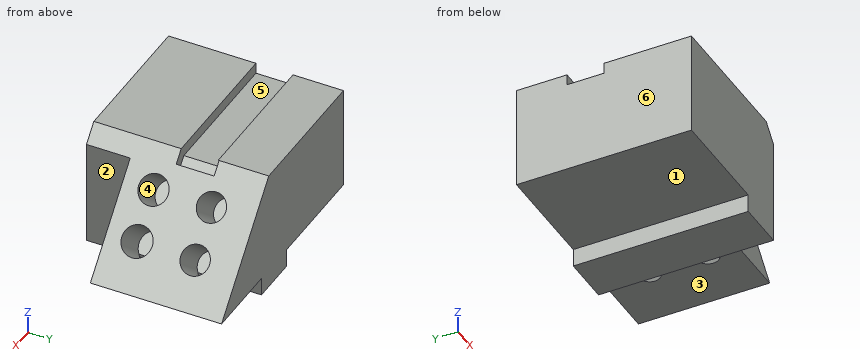
```python
from build123d import *

# Parameters (mm, degrees)
F1_DEPTH = 101.6
F2_W     = 83.0206293613
F2_H     = 21.5133689344
F3_DEPTH = 6.35
F5_DEPTH = 6.35
F4_R     = 8.5928571877
F4_R_2   = 8.3348569543
F4_R_3   = 8.3703398653
F4_R_4   = 8.8433843917
F6_DEPTH = 25.4
F8_DEPTH = 25.4


with BuildPart() as f1:
    # F0 (on Front) → F1 (new body)
    with BuildSketch(Plane.XZ):
        Polygon((29.7097470611, 36.9836613536), (-53.3108823001, 36.9836613536), (-53.3108823001, -23.3776271343), (9.7702555358, -23.3776271343), (9.7702555358, -33.9363776147), (37.8775633872, -33.9363776147), (37.8775633872, -23.3776271343), (82.1659564972, -23.3776271343), align=None)
    extrude(amount=F1_DEPTH)

    # F2 (on face) → F3 (cut)
    with BuildSketch(Plane.XY.offset(36.9836613536)):
        with Locations((-11.8005676195, -40.090886876)):
            Rectangle(F2_W, F2_H)
    extrude(amount=-F3_DEPTH, mode=Mode.SUBTRACT)

    # F4 (on face) → F5 (cut)
    with BuildSketch(Plane(origin=(35.2375904862, 0, 30.6227794812), x_dir=(0, 1, 0), z_dir=(0.7548028054, 0, 0.6559517703))):
        Polygon((-29.3342024088, 8.4272101627), (-50.8475713432, 8.4272101627), (-50.8475713432, 0), (-28.8472529501, 0), (-28.8472529501, 8.4272101627), align=None)
    extrude(amount=-F5_DEPTH, mode=Mode.SUBTRACT)

    # F4 (on face) → F6 (cut)
    with BuildSketch(Plane(origin=(35.2375904862, 0, 30.6227794812), x_dir=(0, 1, 0), z_dir=(0.7548028054, 0, 0.6559517703))):
        with Locations((-58.5515610874, -16.0959567875)):
            Circle(F4_R)
        with Locations((-25.0144358724, -15.7757736742)):
            Circle(F4_R_2)
        with Locations((-24.6950350702, -44.2721843719)):
            Circle(F4_R_3)
        with Locations((-58.5515610874, -43.9519882202)):
            Circle(F4_R_4)
    extrude(amount=-F6_DEPTH, mode=Mode.SUBTRACT)

    # F7 (on face) → F8 (cut)
    with BuildSketch(Plane.XZ.offset(101.6)):
        Polygon((37.8775633872, 27.584966273), (37.8775633872, -23.3776271343), (82.1659564972, -23.3776271343), align=None)
    extrude(amount=-F8_DEPTH, mode=Mode.SUBTRACT)


solid = f1.part
```
Can you work these out from the model? Positions are in its coordinate system, mm. Face numbers are marked on the shaded views. A direction names the side the tool comes from. Coordinates: 2 decimals unless noted, no trailing zeros. Order: outer loops, then holes, each group sorted by start corner. A loop starts at its lowest first (then second) coordinate and runs counter-clockwise, first axis right, second up. Notation, with made-up numbers: (26, 71) -> (53, 71) arc R16 ccw to (53, 81) -> close; hole circle Ø9 at (-31, 15.25). An arc over 180 degrees is marked (long way). Write each question's results on one line, items separated by ' | '.
Item 1: If I drill on line 1 along Y through (x, z) = (30, 28); line 2 along Z through (x, y) = (2.5, -26.5); line 3 along X through (y, z) = (-31, 13), over which ranges is the centre line in solid material (lowest first)?
Results are:
line 1: -101.6 to -50.85, -28.85 to 0 | line 2: -23.38 to 36.98 | line 3: -53.31 to 30.17, 47.85 to 50.55
Item 2: I want a section at A-A, the plane y = -63. Write out the boundary of the cut face in (x, z).
Results are:
outline: (-53.31, -23.38) -> (9.77, -23.38) -> (9.77, -33.94) -> (37.88, -33.94) -> (37.88, -23.38) -> (48.51, -23.38) -> (39.88, -13.44) -> (59.05, 3.22) -> (50.62, 12.92) -> (31.45, -3.74) -> (21.8, 7.36) -> (40.97, 24.02) -> (29.71, 36.98) -> (-53.31, 36.98) -> close; (51.76, -23.38) -> (82.17, -23.38) -> (69.08, -8.32) -> close
Item 3: I'm going to push flat-ended pins straight in: pin 1 Ø12 at (x, z) = (57.5, -2.5) entering from -Y; pin 2 Ø1.5 at (y, z) = (-84, 27) entering from +X; pin 3 Ø2 at (y, z) = (-75, 20) entering from +X. Where does each tip first touch, or does it pass through?
Results are:
pin 1: y = -76.2 | pin 2: x = 37.88 | pin 3: x = 45.34
Item 4: I want a section at B-B, the plane x = -37. Write out the boundary of the cut face in (y, z), then the cut area to 3 significant figures.
Results are:
outline: (-101.6, -23.38) -> (0, -23.38) -> (0, 36.98) -> (-29.33, 36.98) -> (-29.33, 30.63) -> (-50.85, 30.63) -> (-50.85, 36.98) -> (-101.6, 36.98) -> close | area: 6,000 mm²
Item 5: I want a section at C-C, the plane y = -7.5. Write out the boundary of the cut face in (x, z).
Results are:
outline: (-53.31, -23.38) -> (9.77, -23.38) -> (9.77, -33.94) -> (37.88, -33.94) -> (37.88, -23.38) -> (82.17, -23.38) -> (29.71, 36.98) -> (-53.31, 36.98) -> close
Item 6: If we mould it in two halves opening along X, with no side actions, what happens to the marked faces 4, 5 and 6? For each: +X half, -X half, draft (parallel to the pull), parting line (faces both ways), or undercut.
Results are:
face 4: undercut | face 5: draft | face 6: -X half
Item 7: I want a section at D-D, the plane z = 11.5. Count the separate pieces of the cut face and the enclosed holes in it, then the cut area to 3 significant figures.
Results are:
separate pieces: 1 | enclosed holes: 2 | area: 9,640 mm²
Item 8: Which directions (+Z, -Z, +X, -X, +Y, -Y) give clear straight access to the entire face, cutting with the end or side of a thin tool? Please do the marked faces 1, 2 and 3.
Results are:
face 1: -Z, -X, +Y, -Y | face 2: -Z, +X, -Y | face 3: -Z, +X, +Y, -Y
